```python
from build123d import *

# Parameters (mm, degrees)
F0_R     = 7.5
F1_DEPTH = 2
F3_DEPTH = 2


with BuildPart() as f1:
    # F0 (on Top) → F1 (new body)
    with BuildSketch(Plane.XY):
        Circle(F0_R)
    extrude(amount=F1_DEPTH)

    # F2 (on face) → F3 (join)
    with BuildSketch(Plane.XY.offset(2)):
        Polygon((3.580205, 6.186631), (0, 6.182709), (-1.645398, 2.474013), (0, 3.108835), (-2.781395, -1.735857), (-1.211046, -1.20127), (-4.08445, -5.511376), (2.567615, 0), (0.559772, -0.633272), (3.466587, 3.944127), (2.163532, 3.442952), align=None)
    extrude(amount=F3_DEPTH)


solid = f1.part
```
CAD build for the part. Positions are in the model's coordinates, mm. A direction names the side the tool comes from. Give positions to 0.01 mm unless a question says otherwise; leave off trailing zeros. Loops run counter-clockwise (first coordinate to the right, second up) from the corner with the lowest first, then second, coordinate; pieces in that order, holes last. Notation, with made-up numbers: M 4.5,8 L 57.5,8 A24 ccw 57.5,43 Z; hole C 56,-8 d1. An arc over 180 degrees is marked long. Use one line per item in the form item = value.
Item 1: Slice it at B-B (y = -3.5). List the corners of the cut face in (x, z), plus the area to 3 significant figures.
Determined:
outline = M -6.63,0 L 6.63,0 L 6.63,2 L -1.66,2 L -1.66,4 L -2.74,4 L -2.74,2 L -6.63,2 Z
area = 28.7 mm2
Item 2: Which spindle directions (+Z, -Z, +X, -X, +Y, -Y) get a long thin tool onto all of the face, cutting with end or side? Do faces 1 (the face through (-0.8, -2.79, 2.99)), 2 (the face through (-0.811, 4.354, 2.986)), 3 (the face through (2.862, 4.796, 2.986)). Say none if no direction does.
Determined:
face_1 = +Z, +X, -Y
face_2 = +Z, -X, +Y
face_3 = +Z
Item 3: Slice it at D-D (z = 1.55). List the corners of the cut face in (x, y), plus the area to 3 significant figures.
Determined:
outline = C 0,0 d15
area = 177 mm2
Item 4: Slice it at A-A (z = 3.45). List the corners of the cut face in (x, y).
Determined:
outline = M -4.08,-5.51 L 2.57,0 L 0.56,-0.63 L 3.47,3.94 L 2.16,3.44 L 3.58,6.19 L 0,6.18 L -1.65,2.47 L 0,3.11 L -2.78,-1.74 L -1.21,-1.2 Z
Item 5: Flat gauge pin, fed straight in: pin 1 (1 mm diameter, centred on x = 5, z = 0.5, fed in from -Y). Where does the tip first touch, or does it go through?
Determined:
pin_1 = -6
Item 6: Slice it at C-C (x = 6). List the corners of the cut face in (y, z).
Determined:
outline = M -4.5,0 L 4.5,0 L 4.5,2 L -4.5,2 Z
Item 7: Drill centre lines: probe 1 along Z at (x, y) = (-5.5, 1.5); probe 2 along Y at (x, z) = (-3.5, 1.75); probe 3 along Y at (x, z) = (1, 1.05). Where is each one in solid material? Low to high. Write a range as from..to.
Determined:
probe_1 = 0..2
probe_2 = -6.63..6.63
probe_3 = -7.43..7.43
Item 8: Two-plate mould, pull along Y, no slides. Class faces 4 (the face through (2.824, 3.697, 2.986)), 5 (the face through (-7.493, 0.33, 0.986)), 6 (the face through (0, 0, 0)): pulls with the +Y half, pulls with the -Y half, needs draft (parallel to the pull), parting line crosses it, or undercut.
Determined:
face_4 = undercut
face_5 = parting line crosses it
face_6 = needs draft
